Geometry: final body of the model. Coordinates: model frame, mm. A direction names the side the tool comes from. Coordinates: 2 decimals unless noted, no trailing zeros. Loops run counter-clockwise (first coordinate to the right, second up) from the corner with the lowest first, then second, coordinate; pieces in that order, holes last. Notation, with made-up numbers: (59.25, -17.75) -> (70.25, -17.75) arc R19 cw to (70.25, 14.25) -> close; hole circle Ø11 at (-0.5, 85). An arc over 180 degrees is marked (long way). One line per item, written item: value. Start each with the question number.
Item 1: Section query C-C on y = 4.5. Return loops of the section in (x, z).
Item 2: Section query A-A on x = 1.1. Return loops of the section in (y, z), then the cut area to 3 significant figures.
Item 3: Set-up query: faces 4 (the flat face through (1, 13, 0)), 5 (the cylindrical face through (0.76, -0.17, -1.67)), 6 (the flat face through (1, 10, -2)). Return all of +Z, -Z, +X, -X, +Y, -Y with unobstructed straight access to the full face (end or side cutting, diameter ignored); none if empty.
Item 4: Contact query for flat-ended pins moving along their axis: pin 1 Ø0.8 at (x, y) = (1, 12.5) entering from +Z; pin 2 Ø0.8 at (x, z) = (0.5, -4.5) entering from -Y. Output: stop coordinate, or through.
Item 5: Section query B-B on y = 7.5. Return loops of the section in (x, z), then the cut area to 3 significant figures.
Item 6: Mould query, pull axis Z, two halves, no side actions, for faces 1 (the cylindrical face through (0.76, 0.57, -8.4)), 2 (the flat face through (0, 9, -1)), 3 (the cylindrical face through (0.74, 5.57, -2.6)). Classes: +Z half, -Z half, draft (parallel to the pull), parting line (faces both ways), or undercut.
Item 7: Ray query, probe 1 along Y at (x, z) = (1, -7.25); probe 2 along Y at (x, z) = (1.05, -4.5); probe 3 along Z at (x, y) = (0.3, 9.75). Return the intervals inside material, ascending. Write a range as from..to.
Autodesk Inventor part; units mm, degrees
ref_plane "YZ Plane" through (0, 0, 0) normal (1, 0, 0) x (0, 1, 0)
ref_plane "XZ Plane" through (0, 0, 0) normal (0, 1, 0) x (-1, 0, 0)
ref_plane "XY Plane" through (0, 0, 0) normal (0, 0, 1) x (1, 0, 0)
sketch "スケッチ1" plane through (0, 0, 0) normal (1, 0, 0) x (0, 1, 0)
  line L0 (20, 0) -> (0, 0)
  line L1 (0, 0) -> (0, -9)
  line L2 (0, -9) -> (20, -9)
  line L3 (20, -9) -> (20, 0)
  circle A0 centre (2, 2) radius 2
  circle A1 centre (2, 2) radius 0.8
  line L4 (4, 4) -> (0, 4)
  line L5 (0, 4) -> (0, 0)
  line L6 (0, 0) -> (4, 0)
  line L7 (4, 0) -> (4, 4)
  circle A2 centre (2, 2) radius 4
  point P0 (4, 2)
  point P1 (0, 2)
  point P2 (5.4641, 0)
  point P3 (0, -1.4641)
  dimension "d0" = 4
  dimension "d1" = 1.6
  dimension "d2" = 9
  dimension "d3" = 20
  dimension "d12" = 8
extrude "押し出し1" add sketch "スケッチ1" along normal blind 1.5
fillet "フィレット1" radius 2 5 edges at (0.75, 20, 0) (0.75, 20, -9) (0.75, 0, -9) (0.75, 0, -1.4641) (0.75, 5.4641, 0)
sketch "スケッチ2" plane through (1.5, 0, 0) normal (1, 0, 0) x (0, 0, -1)
  circle A0 centre (2, 18) radius 0.8
  circle A1 centre (7, 18) radius 0.8
  circle A2 centre (7, 2) radius 0.8
  arc A3 (9, 18) -> (7, 20) centre (7, 18) ccw
  arc A4 (2, 20) -> (0, 18) centre (2, 18) ccw
  arc A5 (7, 0) -> (9, 2) centre (7, 2) ccw
  line L0 (2, 18) -> (7, 18) construction
  line L1 (7, 18) -> (7, 2) construction
  line L2 (7, 2) -> (2, 2) construction
  line L3 (2, 2) -> (2, 18) construction
  line L4 (2, 15) -> (7, 15)
  line L5 (7, 15) -> (7, 5)
  line L6 (7, 5) -> (2, 5)
  line L7 (2, 5) -> (2, 15)
  point P0 (0, 0)
  dimension "d6" = 1.6
  dimension "d7" = 1.6
  dimension "d8" = 1.6
  dimension "d13" = 3
  dimension "d14" = 3
extrude "押し出し2" cut sketch "スケッチ2" against normal through all
fillet "フィレット2" radius 2 4 edges at (0.75, 15, -2) (0.75, 15, -7) (0.75, 5, -7) (0.75, 5, -2)
properties part number "chest_cover_side_joint"
Reply:
1. outline: (0, -9) -> (1.5, -9) -> (1.5, 5.12) -> (0, 5.12) -> close
2. outline: (-0.67, -0.98) arc R2 cw to (0, -2.47) -> (0, -7) arc R2 ccw to (2, -9) -> (18, -9) arc R2 ccw to (20, -7) -> (20, -2) arc R2 ccw to (18, 0) -> (8, 0) arc R2 cw to (6, 2) arc R4 ccw (long way) to start; hole circle Ø1.6 at (2, -7); hole circle Ø1.6 at (2, 2); hole (5, -5) arc R2 ccw to (7, -7) -> (13, -7) arc R2 ccw to (15, -5) -> (15, -4) arc R2 ccw to (13, -2) -> (7, -2) arc R2 ccw to (5, -4) -> close; hole circle Ø1.6 at (18, -7); hole circle Ø1.6 at (18, -2)
2. area: 166 mm²
3. face 4: +Z, +X, -X, +Y
3. face 5: -Z, +X, -X, -Y
3. face 6: +X, -X
4. pin 1: stops at z = 0
4. pin 2: stops at y = 0
5. outline: (0, -9) -> (1.5, -9) -> (1.5, -7) -> (0, -7) -> close; (0, -2) -> (1.5, -2) -> (1.5, 0.06) -> (0, 0.06) -> close
5. area: 6.10 mm²
6. face 1: -Z half
6. face 2: draft
6. face 3: undercut
7. probe 1: y = 0.02..1.24, 2.76..17.24, 18.76..19.98
7. probe 2: y = 0..5, 15..20
7. probe 3: z = -9..-7, -2..0
